The figure shows three views and two pictorial views of one solid part (mm, origin at its lowest corner). Answer the questions. Coordinates: 2 decimals unless noted, no trailing zeros. Order: outer loops, then holes, each group sorted by start corner. A loop starts at its lowest first (then second) coordinate and runs counter-clockwise, first axis right, second up. Notation, with made-up numbers: M -23,60.25 L -15,60.25 A22 cw -15,84.25 Z; hole C 13.5,-31.75 d1. An arc over 180 degrees is marked long. Answer in a Markdown table with one row per item. Add a question column.
Item 1: Flat-ended cylindrical pins translate along their axes: pin 1 Ø1.2 at (y, z) = (22.5, 4) entering from -X; pin 2 Ø0.9 at (x, y) = (8, 33) entering from +Z; pin 3 Ø3 at (y, z) = (35.5, 4) entering from -X; pin 4 Ø3 at (y, z) = (29.5, 5) entering from +X. Find the tip coordinate at first contact, or state that the pin passes through.
Item 2: The mould has two halves that part along X. Classify the marked faces 1 and 2: released by +X, released by -X, zero draft, split by the parting line, or undercut.
Item 3: The part is cut by section A-A (y = 35). Write down the section's boundary in (x, z), then the cut area to 4 significant figures.
Item 4: The part is cut by section C-C (z = 1.15). Write down the section's boundary in (x, y), then the cut area to 3 significant figures.
Item 5: The part is cut by section D-D (y = 24.5). Write down the section's boundary in (x, z), then the cut area to 3 significant figures.
Item 6: The part is cut by section B-B (x = 5). Write down the section's boundary in (y, z).
Item 7: Consider line 1 (Y direction, x = 5, z = 2.2); line 2 (X direction, y = 43.5, z = 5.25); line 3 (Z direction, x = 2.75, y = 25). Determine where each line is inside the solid, lowest interval first. Write a range as from..to.
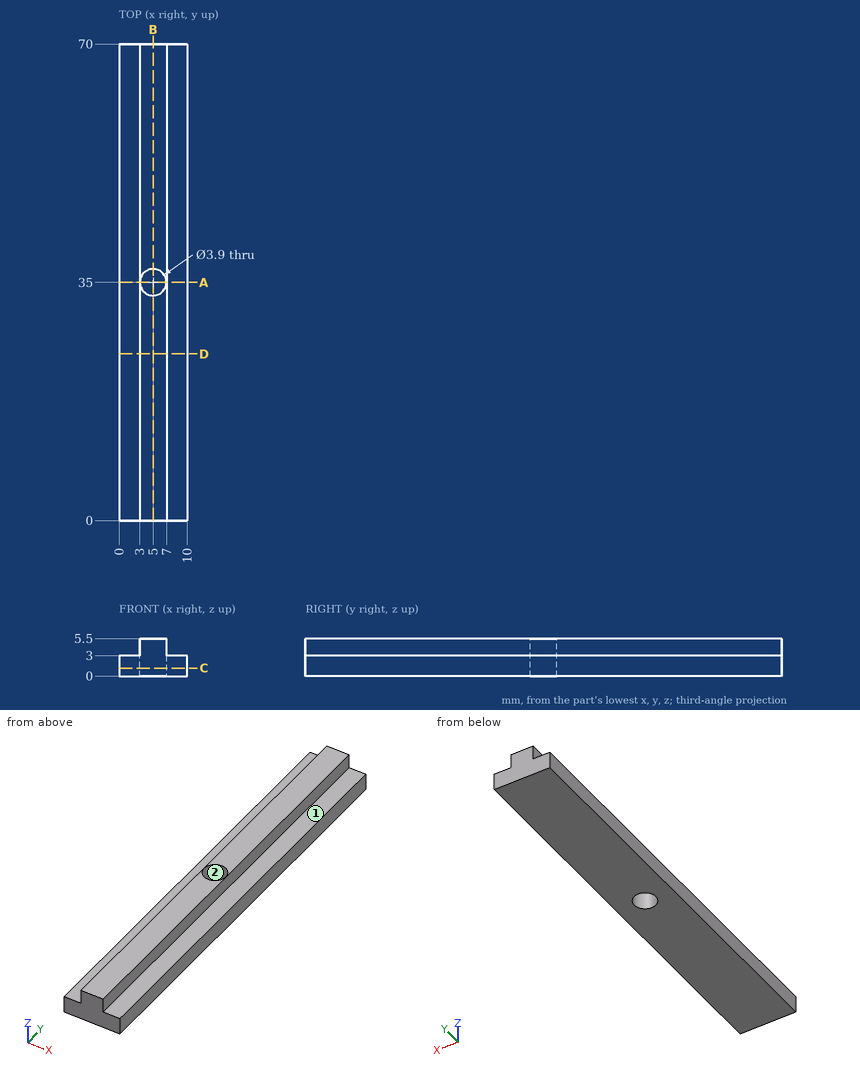
Reply:
| question | item | result |
|---|---|---|
| 1 | pin 1 | stops at x = 3 |
| 1 | pin 2 | stops at z = 3 |
| 1 | pin 3 | stops at x = 0 |
| 1 | pin 4 | stops at x = 7 |
| 2 | face 1 | zero draft |
| 2 | face 2 | undercut |
| 3 | outline | M 0,0 L 3.05,0 L 3.05,5.5 L 3,5.5 L 3,3 L 0,3 Z; M 6.95,0 L 10,0 L 10,3 L 7,3 L 7,5.5 L 6.95,5.5 Z |
| 3 | area | 18.55 mm2 |
| 4 | outline | M 0,0 L 10,0 L 10,70 L 0,70 Z; hole C 5,35 d3.9 |
| 4 | area | 688 mm2 |
| 5 | outline | M 0,0 L 10,0 L 10,3 L 7,3 L 7,5.5 L 3,5.5 L 3,3 L 0,3 Z |
| 5 | area | 40.0 mm2 |
| 6 | outline | M 0,0 L 33.05,0 L 33.05,5.5 L 0,5.5 Z; M 36.95,0 L 70,0 L 70,5.5 L 36.95,5.5 Z |
| 7 | line 1 | y = 0..33.05, 36.95..70 |
| 7 | line 2 | x = 3..7 |
| 7 | line 3 | z = 0..3 |
